Design review of the part built by this model. Coordinates are the model's own, in mm. A direction names the side the tool comes from. Round coordinates to 2 decimals unless told otherwise and drop trailing zeros. Order: outer loops, then holes, each group sorted by start corner. A loop starts at its lowest first (then second) coordinate and runs counter-clockwise, first axis right, second up. Notation, with made-up numbers: M 41.25,13.25 L 48.25,13.25 A13 cw 48.25,35.25 Z; hole C -23,-25 d3. An arc over 180 degrees is marked long. Write item = value, one per line. Start each with the question number.
```python
from build123d import *

# Parameters (mm, degrees)
BOSS_EXTRUDE1_DEPTH   = 38.1
SKETCH5_W             = 7.62
SKETCH5_H             = 3.175
BOSS_EXTRUDE2_DEPTH   = 10.16
F_6_CLEARANCE_HOLE1_D = 3.7973
BOSS_EXTRUDE3_DEPTH   = 3.175
FILLET1_R             = 6.35
FILLET2_R             = 2.54
FILLET3_R             = 2.54
FILLET4_R             = 2.54
BOSS_EXTRUDE6_DEPTH   = 6.35
CUT_EXTRUDE1_REACH    = 86.541
SKETCH19_W            = 1.27
SKETCH19_H            = 3.048


with BuildPart() as part:
    # Sketch1 → Boss-Extrude1 (new body)
    with BuildSketch(Plane(origin=(0, 0, 0), x_dir=(1, 0, 0), z_dir=(0, 1, 0))):
        Polygon((-34.925, -15.875), (34.925, -15.875), (34.925, 15.875), (34.925, 28.575), (28.575, 28.575), (28.575, 15.875), (28.575, -9.525), (-28.575, -9.525), (-28.575, 15.875), (-34.925, 15.875), align=None)
    extrude(amount=BOSS_EXTRUDE1_DEPTH)

    # Sketch5 → Boss-Extrude2 (add)
    with BuildSketch(Plane(origin=(-28.575, 0, 0), x_dir=(0, 0, -1), z_dir=(1, 0, 0))):
        with Locations((4.445, 18.0975)):
            Rectangle(SKETCH5_W, SKETCH5_H)
    boss_extrude2 = extrude(amount=BOSS_EXTRUDE2_DEPTH)

    # #6 Clearance Hole1 (through all)
    with Locations(Plane(origin=(0, 19.685, 0), x_dir=(1, 0, 0), z_dir=(0, 1, 0))):
        with Locations((-23.241, 4.445)):
            f_6_clearance_hole1 = Hole(F_6_CLEARANCE_HOLE1_D / 2)

    # Mirror4: Boss-Extrude2, #6 Clearance Hole1 across plane
    add(boss_extrude2.mirror(Plane(origin=(0, 0, 0), x_dir=(0, 0, 1), z_dir=(1, 0, 0))))
    add(f_6_clearance_hole1.mirror(Plane(origin=(0, 0, 0), x_dir=(0, 0, 1), z_dir=(1, 0, 0))), mode=Mode.SUBTRACT)

    # Sketch11 → Boss-Extrude3 (add)
    with BuildSketch(Plane.XZ):
        Polygon((-28.575, -28.575), (-28.575, 9.525), (28.575, 9.525), (28.575, -28.575), (34.925, -28.575), (34.925, 15.875), (-34.925, 15.875), (-34.925, -28.575), align=None)
    extrude(amount=BOSS_EXTRUDE3_DEPTH)

    # Fillet1
    fillet1_edges = [part.edges().sort_by_distance(p)[0] for p in [
        (34.925, 17.4625, 15.875),
        (-34.925, 17.4625, 15.875),
    ]]
    fillet(fillet1_edges, radius=FILLET1_R)

    # Fillet2
    fillet2_edges = [part.edges().sort_by_distance(p)[0] for p in [
        (-28.575, 18.0975, -8.255),
        (-28.575, 18.0975, -0.635),
        (28.575, 18.0975, -0.635),
        (28.575, 18.0975, -8.255),
    ]]
    fillet(fillet2_edges, radius=FILLET2_R)

    # Fillet3
    fillet3_edges = [part.edges().sort_by_distance(p)[0] for p in [
        (-28.575, 16.51, -4.445),
        (28.575, 16.51, -4.445),
    ]]
    fillet(fillet3_edges, radius=FILLET3_R)

    # Fillet4
    fillet4_edges = [part.edges().sort_by_distance(p)[0] for p in [
        (-28.575, 17.4625, 9.525),
        (28.575, 17.4625, 9.525),
    ]]
    fillet(fillet4_edges, radius=FILLET4_R)

    # Sketch18 → Boss-Extrude6 (add)
    with BuildSketch(Plane.ZY.offset(34.925)):
        Polygon((-24.511, 19.05), (-28.575, 19.05), (-28.575, 0), (-15.875, 0), (-15.875, 6.35), (-24.511, 6.35), align=None)
    extrude(amount=-BOSS_EXTRUDE6_DEPTH)

    # Sketch19 → Cut-Extrude1 (cut, up to next)
    with BuildSketch(Plane.ZY.offset(34.925), mode=Mode.PRIVATE) as cut_extrude1_sk1:
        with Locations((-15.24, 16.129)):
            Rectangle(SKETCH19_W, SKETCH19_H)
    cut_extrude1_tool1 = extrude(cut_extrude1_sk1.sketch, amount=-CUT_EXTRUDE1_REACH, mode=Mode.PRIVATE) & part.part
    # Sketch19 → Cut-Extrude1 (cut, up to next)
    with BuildSketch(Plane.ZY.offset(34.925), mode=Mode.PRIVATE) as cut_extrude1_sk2:
        with Locations((-25.146, 16.129)):
            Rectangle(SKETCH19_W, SKETCH19_H)
    cut_extrude1_tool2 = extrude(cut_extrude1_sk2.sketch, amount=-CUT_EXTRUDE1_REACH, mode=Mode.PRIVATE) & part.part
    add(cut_extrude1_tool1.solids().sort_by_distance((-34.925, 16.129, -15.24))[0], mode=Mode.SUBTRACT)
    add(cut_extrude1_tool2.solids().sort_by_distance((-34.925, 16.129, -25.146))[0], mode=Mode.SUBTRACT)


solid = part.part
```
(1) Consider section A-A, the plane x = -20. Write out the cut boundary in (y, z) (3 decimals).
(2) Consider section B-B, the plane z = 3.5. Write out the cut boundary in (x, y) (3 decimals).
(3) For faces 1 (the face through (21, 16.51, -4)), 2 (the face through (-32, 18, -24.511)), 3 (the face through (-18.415, 18, -4)), list the 3-axis set-ups (+Z, -Z, +X, -X, +Y, -Y) from which the entire face can be reached by the end or side of a thin tool; tool diameter is ignored.
(4) Insertion check: pin 1 (20.5 mm diameter, centred on x = -9.5, y = 21.5, fed in from -Z) (3 decimals); pin 2 (8 mm diameter, centred on x = 23, z = -6.5, fed in from +Y) (3 decimals); pin 3 (4.5 mm diameter, centred on x = 23.241, z = -4.445, fed in from -Y). Each pin has a flat end and moves straight along its axis. Give the tip position at first contact, or say it passes through.
(5) For line 1 along X through (y, z) = (3.5, -20) (3 decimals); line 2 along Z through (x, y) = (-20, 26) (3 decimals); line 3 along Z through (x, y) = (-31, 19) (3 decimals), list the stretches that pass through material, from the lowest coordinate up. Write a range as [from, to].
(6) Draft analysis for pull direction Z (two halves, no side actions). For faces 4 (the face through (22, 18, -0.635)), 5 (the face through (-32, 10, -24.511)), 6 (the face through (-32, 8, -28.575)), 7 (the face through (-21, 16.51, -4)), state which applies: pulls with the +Z half, pulls with the -Z half, needs draft (parallel to the pull), parting line crosses it, or undercut.
(7) Consider section C-C, the plane y = 8. Write out the cut boundary in (x, z) (3 decimals).
(8) Consider section D-D, the plane y = 25. Write out the cut boundary in (x, z) (3 decimals), then the cut area to 3 significant figures.
Completed:
q1.outline = M -3.175,9.525 L 38.1,9.525 L 38.1,15.875 L -3.175,15.875 Z; M 16.51,-8.255 L 19.685,-8.255 L 19.685,-0.635 L 16.51,-0.635 Z
q2.outline = M -34.925,-3.175 L -28.575,-3.175 L -28.575,38.1 L -34.925,38.1 Z; M 28.575,-3.175 L 34.925,-3.175 L 34.925,38.1 L 28.575,38.1 Z
q3.face_1 = -Z, -Y
q3.face_2 = -X, +Y
q3.face_3 = -Z, +Y, -Y
q4.pin_1 = -8.255
q4.pin_2 = 19.685
q4.pin_3 = 16.51
q5.line_1 = [-34.925, -28.575], [28.575, 34.925]
q5.line_2 = [9.525, 15.875]
q5.line_3 = [-28.575, -24.511], [-15.875, 15.394]
q6.face_4 = undercut
q6.face_5 = undercut
q6.face_6 = pulls with the -Z half
q6.face_7 = needs draft
q7.outline = M -34.925,-28.575 L -28.575,-28.575 L -28.575,-24.511 L -34.925,-24.511 Z; M -34.925,-15.875 L -28.575,-15.875 L -28.575,6.985 A2.54 cw -26.035,9.525 L 26.035,9.525 A2.54 cw 28.575,6.985 L 28.575,-28.575 L 34.925,-28.575 L 34.925,9.525 A6.35 ccw 28.575,15.875 L -28.575,15.875 A6.35 ccw -34.925,9.525 Z
q8.outline = M -34.925,-15.875 L -28.575,-15.875 L -28.575,6.985 A2.54 cw -26.035,9.525 L 26.035,9.525 A2.54 cw 28.575,6.985 L 28.575,-28.575 L 34.925,-28.575 L 34.925,9.525 A6.35 ccw 28.575,15.875 L -28.575,15.875 A6.35 ccw -34.925,9.525 Z
q8.area = 832 mm2
